Autodesk Inventor part; units mm, degrees
ref_plane "Work Plane1" through (0, 0, 1.25) normal (0, 0, -1) x (-1, 0, 0)
ref_plane "Work Plane2" through (0, 0, 0.75) normal (0, 0, -1) x (-1, 0, 0)
ref_plane "Work Plane3" through (0, 0, 0.45) normal (0, 0, -1) x (-1, 0, 0)
sketch "Sketch1" plane through (0, 0, 0) normal (0, 0, 1) x (1, 0, 0)
  line L0 (-25, 1.25) -> (-25, -0.25)
  line L1 (-24, -1.25) -> (24, -1.25)
  line L2 (25, -0.25) -> (25, 1.25)
  line L3 (25, 1.25) -> (-25, 1.25)
  line L4 (0, 0) -> (0, 5.9906) construction
  line L5 (0, 0) -> (2.2727, 0) construction
  arc A0 (-17.775, 1.25) -> (-13.725, 1.25) centre (-15.75, 1.25) ccw
  arc A1 (-13.275, 1.25) -> (-9.225, 1.25) centre (-11.25, 1.25) ccw
  arc A2 (-8.775, 1.25) -> (-4.725, 1.25) centre (-6.75, 1.25) ccw
  arc A3 (-4.255, 1.25) -> (-2.535, 1.25) centre (-3.395, 1.25) ccw
  arc A4 (-1.965, 1.25) -> (-0.245, 1.25) centre (-1.105, 1.25) ccw
  arc A5 (0.225, 1.25) -> (4.275, 1.25) centre (2.25, 1.25) ccw
  arc A6 (4.725, 1.25) -> (8.775, 1.25) centre (6.75, 1.25) ccw
  arc A7 (9.225, 1.25) -> (13.275, 1.25) centre (11.25, 1.25) ccw
  arc A8 (13.725, 1.25) -> (17.775, 1.25) centre (15.75, 1.25) ccw
  arc A9 (18.925, 1.25) -> (20.675, 1.25) centre (19.8, 1.25) ccw
  arc A10 (21.625, 1.25) -> (23.375, 1.25) centre (22.5, 1.25) ccw
  arc A11 (-25, -0.25) -> (-24, -1.25) centre (-24, -0.25) ccw
  arc A12 (24, -1.25) -> (25, -0.25) centre (24, -0.25) ccw
  arc A13 (-22.275, 1.25) -> (-18.225, 1.25) centre (-20.25, 1.25) ccw
  point P0 (-25, -1.25)
  point P1 (25, -1.25)
  dimension "d0" = 2.5
  dimension "d1" = 50
  dimension "d2" = 90
  dimension "d4" = 4.05
  dimension "d5" = 4.05
  dimension "d6" = 4.05
  dimension "d7" = 1.72
  dimension "d8" = 1.72
  dimension "d9" = 4.05
  dimension "d10" = 4.05
  dimension "d11" = 4.05
  dimension "d12" = 4.05
  dimension "d13" = 1.75
  dimension "d14" = 1.75
  dimension "d16" = 4.5
  dimension "d17" = 4.5
  dimension "d18" = 3.355
  dimension "d19" = 2.29
  dimension "d20" = 3.355
  dimension "d21" = 4.5
  dimension "d22" = 4.5
  dimension "d23" = 4.5
  dimension "d25" = 2.7
  dimension "d26" = 1
  dimension "d51" = 2.5
  dimension "d52" = 4.05
  dimension "d53" = 4.5
  dimension "d101" = 4.05
extrude "Extrusion1" add sketch "Sketch1" along normal blind 12 contours L3 A13 A0 A1 A2 A3 A4 A5 A6 A7 A8 A9 A10 L2 A12 L1 A11 L0
sketch "Sketch2" plane through (-24, -1.25, 0) normal (0, -1, 0) x (1, 0, 0)
  line L0 (49, 0) -> (49, 12)
  line L1 (-1, 0) -> (-1, 12)
  line L2 (0, 0) -> (48, 0)
  line L3 (-0.714, 0.4) -> (48.714, 0.4)
  line L4 (48.714, 1) -> (-0.714, 1)
  line L5 (48.714, 5) -> (-0.714, 5)
  line L6 (-0.714, 5) -> (-0.714, 5.6)
  line L7 (-0.714, 5.6) -> (48.714, 5.6)
  line L8 (48.714, 5.6) -> (48.714, 5)
  line L9 (-0.714, 1) -> (-0.714, 0.4)
  line L10 (48.714, 1) -> (48.714, 0.4)
  point P0 (24, 0)
  point P1 (37.5, 3)
  point P2 (15, 3)
  point P3 (48.714, 5.3)
  dimension "d29" = 11.5
  dimension "d30" = 22.5
  dimension "d32" = 3
  dimension "d33" = 0.6
  dimension "d34" = 0.6
  dimension "d35" = 0.4
  dimension "d36" = 4
  dimension "d48" = 0.286
  dimension "d49" = 0.6
  dimension "d50" = 0.286
hole "Hole1" at (13.5, -1.25, 3) at (-9, -1.25, 3) direction (0, 1, 0) diameter 1.5 end through all
extrude "Extrusion3" cut sketch "Sketch2" against normal blind 0.3
sketch "Sketch3" plane through (0, 0, 0) normal (0, 0, -1) x (-1, 0, 0)
  line L0 (-23, 1.25) -> (-1.5933, 1.25)
  line L1 (-1.5933, 1.25) -> (-1.5933, 1.075)
  line L2 (-1.5933, 1.075) -> (-23, 1.075)
  line L3 (-23, 1.075) -> (-23, 1.25)
  line L4 (7.4905, 1.25) -> (21.4905, 1.25)
  line L5 (21.4905, 1.25) -> (21.4905, 1.075)
  line L6 (21.4905, 1.075) -> (7.4905, 1.075)
  line L7 (7.4905, 1.075) -> (7.4905, 1.25)
  line L8 (8.775, 1.25) -> (9.225, 1.25)
  line L9 (-25, -0.25) -> (-25, 1.25)
  line L10 (25, 1.25) -> (25, -0.25)
  point P0 (0, 0)
  point P1 (9, 1.25)
  dimension "d54" = 0.175
  dimension "d55" = 0.175
  dimension "d56" = 14
  dimension "d57" = 21.4067
  dimension "d58" = 2
  dimension "d59" = 3.5095
extrude "Extrusion4" cut sketch "Sketch3" against normal blind 25.3
ref_plane "Work Plane1" through (0, 0, 1.25) normal (0, 0, -1) x (-1, 0, 0)
sketch "Sketch5" plane through (-24, -1.25, 12) normal (0, -1, 0) x (1, 0, 0)
  circle A0 centre (-2.4, -2.0003) radius 2
  circle A1 centre (50.4, -2.0003) radius 2
  line L0 (-1, -12) -> (-1, 0)
  line L1 (-1, 0) -> (-1, -0.572)
  line L2 (49, -12) -> (49, 0)
  line L3 (49, 0) -> (49, -0.572)
  point P0 (24, -12)
  dimension "d71" = 4
  dimension "d72" = 4
  dimension "d73" = 0.572
  dimension "d74" = 0.572
  dimension "d75" = 1.4
  dimension "d76" = 1.4
extrude "Extrusion6" cut sketch "Sketch5" against normal blind 4
ref_plane "Work Plane2" through (0, 0, 0.75) normal (0, 0, -1) x (-1, 0, 0)
sketch "Sketch6" plane through (0, 0, 0.75) normal (0, 0, -1) x (-1, 0, 0)
  line L0 (-25, 1.25) -> (-23.375, 1.25)
  line L1 (-25, 1.25) -> (-24.4, 1.25)
  line L2 (-24.4, 1.25) -> (-24.4, 0.5)
  line L3 (-24.4, 0.5) -> (-24.124, 0.5)
  line L4 (-24.124, 0.5) -> (-24.4667, -0.2996)
  line L5 (-24.124, 0.5) -> (-23.254, 0.5) construction
  line L6 (-24.4667, -0.2996) -> (-24.9987, -0.2996)
  line L7 (-24.4667, -0.2996) -> (-24.4, -0.2996) construction
  line L8 (-25, 1.25) -> (-25, -0.25)
  line L9 (-25, -0.25) -> (-25, 1.25)
  line L10 (-25, 1.25) -> (-25, -0.25)
  line L11 (-24.4, -0.2996) -> (-24.365, -0.2996)
  arc A0 (-24.714, -0.9501) -> (-24, -1.25) centre (-24, -0.25) ccw
  arc A1 (-25, -0.25) -> (-24.9987, -0.2996) centre (-24.0293, -0.25) ccw
  point P0 (0, 0)
  dimension "d80" = 0.6
  dimension "d81" = 0.75
  dimension "d82" = 0.276
  dimension "d83" = 113.2
  dimension "d84" = 0.87
  dimension "d86" = 0.532
  dimension "d87" = 180
extrude "Extrusion7" cut sketch "Sketch6" against normal blind 6.1
ref_plane "Work Plane3" through (0, 0, 0.45) normal (0, 0, -1) x (-1, 0, 0)
sketch "Sketch7" plane through (0, 0, 0.45) normal (0, 0, -1) x (-1, 0, 0)
  line L0 (-25, 1.25) -> (-24.25, 1.25)
  line L1 (-25, 1.25) -> (-24.4, 1.25)
  line L2 (-24.4, 1.25) -> (-24.4, 0.5)
  line L3 (-24.4, 0.5) -> (-24.124, 0.5)
  line L4 (-24.124, 0.5) -> (-24.4667, -0.2996)
  line L5 (-24.124, 0.5) -> (-23.254, 0.5) construction
  line L6 (-24.4667, -0.2996) -> (-24.9987, -0.2996)
  line L7 (-24.4667, -0.2996) -> (-24.4, -0.2996) construction
  line L8 (-25, 1.25) -> (-25, -0.25)
  line L9 (-25, -0.25) -> (-25, 1.25)
  line L10 (-25, 1.25) -> (-25, -0.25)
  line L11 (-24.4, -0.2996) -> (-24.365, -0.2996)
  arc A0 (-24.714, -0.9501) -> (-24, -1.25) centre (-24, -0.25) ccw
  arc A1 (-25, -0.25) -> (-24.9987, -0.2996) centre (-24.0293, -0.25) ccw
  line L12 (0, 0) -> (0, -6.4481) construction
  line L13 (25, 1.25) -> (24.25, 1.25)
  line L14 (24.4, 1.25) -> (24.4, 0.5)
  line L15 (24.4, 0.5) -> (24.124, 0.5)
  line L16 (24.124, 0.5) -> (23.254, 0.5) construction
  line L17 (24.4, -0.2996) -> (24.365, -0.2996)
  line L18 (24.4667, -0.2996) -> (24.4, -0.2996) construction
  line L19 (24.124, 0.5) -> (24.4667, -0.2996)
  line L20 (24.4667, -0.2996) -> (24.9987, -0.2996)
  arc A2 (24.9987, -0.2996) -> (25, -0.25) centre (24.0293, -0.25) ccw
  line L21 (25, 1.25) -> (25, -0.25)
  line L22 (25, 1.25) -> (25, -0.25)
  line L23 (25, -0.25) -> (25, 1.25)
  line L24 (25, 1.25) -> (24.4, 1.25)
  point P0 (24, -0.25)
  point P1 (24, -0.25)
  dimension "d92" = 0.6
  dimension "d93" = 0.75
  dimension "d94" = 0.276
  dimension "d95" = 113.2
  dimension "d96" = 0.87
  dimension "d97" = 0.532
  dimension "d98" = 180
extrude "Extrusion8" cut sketch "Sketch7" against normal blind 6.1 contours L21 A2 L20 L19 L15 L14 L13
properties part number "3d_LM - Pinza 4" material "PA12 SLS 3D Print"
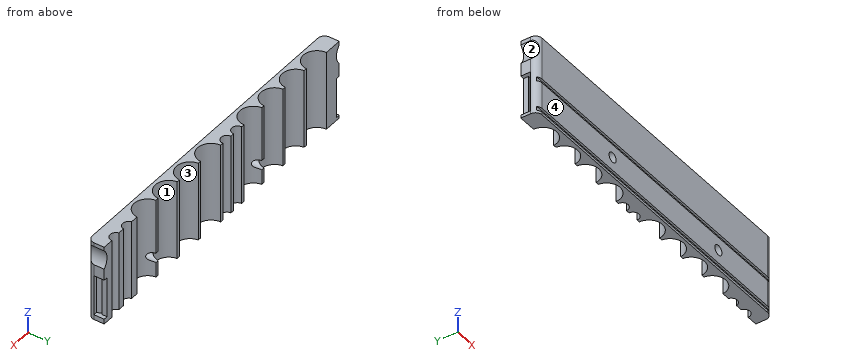
Design review of the part built by this model. Coordinates are the model's own, in mm. Face numbers are marked on the shaded views. Round coordinates to 2 decimals unless told otherwise and drop trailing zeros. Order: outer loops, then holes, each group sorted by start corner. A loop starts at its lowest first (then second) coordinate and runs counter-clockwise, first axis right, second up. Notation, with made-up numbers: M 3,86.25 L 62,86.25 A27 cw 62,119.25 Z; hole C 55,-36.75 d6. An arc over 180 degrees is marked long. Answer as CSV lines item,"result". Start each with the question number.
1) Add section B-B (z = 3). Give the number of separate pieces and of enclosed holes in the cut face, then the cut area to 3 significant figures.
2) Wall thickness on line 1 along Z through (x, y) = (13.5, 0.4); line 2 along Y through (x, z) = (-14, 3.5); line 3 along X through (y, z) = (-1.1, 9.5): over which ranges is each line inside the solid? List them lowest first. Write a range as [from, to].
3) The part is to be moulded in two halves that separate along X. For the marked faces 1, 2, 3 and 4, say which applies: +X half, -X half, draft (parallel to the pull), parting line (faces both ways), or undercut.
4) Add section A-A (x = -6.75). Give the boundary of the cut face in (y, z) (3 decimals).
5) Add section D-D (x = -16.5). Give the boundary of the cut face in (y, z).
6) For pin 1 Ø0.8 at (x, z) = (21, 4.5) entering from +Y (3 decimals), flat-tipped, find the tip position at first contact; note if it passes through.
Resolved:
1,separate pieces,"3"
1,enclosed holes,"0"
1,area,"60.1 mm^2"
2,line 1,"[0, 2.25], [3.75, 12]"
2,line 2,"[-1.25, 0.23]"
2,line 3,"[-24.46, 24.46]"
3,face 1,"undercut"
3,face 2,"-X half"
3,face 3,"undercut"
3,face 4,"draft"
4,outline,"M -1.25,0 L -0.775,0 L -0.775,12 L -1.25,12 L -1.25,5.6 L -0.95,5.6 L -0.95,5 L -1.25,5 L -1.25,1 L -0.95,1 L -0.95,0.4 L -1.25,0.4 Z"
5,outline,"M -1.25,0 L -0.63,0 L -0.63,12 L -1.25,12 L -1.25,5.6 L -0.95,5.6 L -0.95,5 L -1.25,5 L -1.25,1 L -0.95,1 L -0.95,0.4 L -1.25,0.4 Z"
6,pin 1,"y = 1.075"
